Autodesk Inventor part; units mm, degrees
ref_plane "YZ Plane" through (0, 0, 0) normal (1, 0, 0) x (0, 1, 0)
ref_plane "XZ Plane" through (0, 0, 0) normal (0, 1, 0) x (-1, 0, 0)
ref_plane "XY Plane" through (0, 0, 0) normal (0, 0, 1) x (1, 0, 0)
sketch "Sketch1" plane through (0, 0, 0) normal (0, 1, 0) x (-1, 0, 0)
  line L0 (0, 0) -> (1.8, 0)
  line L1 (0, 0) -> (-1.8, 0)
  circle A0 centre (0, 0) radius 2.7
  line L2 (1.8, 0) -> (1.8, 2.0125)
  line L3 (1.8, 0) -> (1.8, -2.0125)
  line L4 (-1.8, 0) -> (-1.8, -2.0125)
  line L5 (-1.8, 0) -> (-1.8, 2.0125)
  circle A1 centre (0, 0) radius 4.7
  dimension "d0" = 1.8
  dimension "d1" = 1.8
  dimension "d2" = 5.4
  dimension "d7" = 9.4
extrude "Extrusion1" add sketch "Sketch1" along normal blind 4 contours L1 L5 A0 L2 L0 | L0 L3 A0 L4 L1 | L2 A0 L3 | L4 A0 L5
extrude "Extrusion2" add sketch "Sketch1" along normal blind 5 from surface at 4 contours L1 L5 A0 L2 L0 | L0 L3 A0 L4 L1
extrude "Extrusion3" add sketch "Sketch1" against normal blind 2 contours L1 L5 A0 L2 L0 | L0 L3 A0 L4 L1 | L2 A0 L3 | L4 A0 L5 | A1
chamfer "Chamfer1" distance 2 angle 45 1 edges at (4.7, 0, 0)
properties part number "driven gear axle"
The listing builds one solid part. Answer for the finished solid, in the listing's coordinates (mm). A direction names the side the tool comes from. Round coordinates to 2 decimals unless told otherwise and drop trailing zeros. Loops run counter-clockwise (first coordinate to the right, second up) from the corner with the lowest first, then second, coordinate; pieces in that order, holes last.
Q1. Find the intervals of material crossed by line 1 (Y direction, x = 2.5, z = -0.5); line 2 (X direction, y = 7, z = -0.5); line 3 (Z direction, x = 0.75, y = 1), in increasing order.
Q2. For a pull along Z with two mould halves and no side action, classify faces 1 (the face through (-2.575, 3.437, -0.811)), 2 (the face through (0, -2, 0)) as released by +Z, released by -Z, zero draft, split by the parting line, or undercut.
Q3. Which of the six approach directions +Z, -Z, +X, -X, +Y, -Y give full straight-line access (tool end or side, diameter ignored) to faces 3 (the face through (1.8, 6, 0)), 4 (the face through (-2, 4, 0)), 5 (the face through (0.613, -0.125, 2.758))?
Q4. Given pin 1 Ø4 at (y, z) = (2, 3.5) entering from -X (3 decimals); pin 2 Ø4.5 at (y, z) = (5.5, 1) entering from -X; pin 3 Ø1.5 at (y, z) = (7.5, 3) entering from -X, each flat-ended and moving along its own axis, determine where each tip first touches the part or whether it passes through.
Q5. Section C-C, the plane y = 1.25 is taken. Determine the outline of the cut face in (x, z), then the cut area to 3 significant figures.
Q6. Section D-D, the plane y = -0.25 is taken. Determine the outline of the cut face in (x, z).
Completed:
1. line 1: y = -2 to 4
1. line 2: x = -1.8 to 1.8
1. line 3: z = -2.59 to 2.59
2. face 1: split by the parting line
2. face 2: zero draft
3. face 3: +Z, -Z, +X, +Y
3. face 4: +Z, -Z, -X, +Y
3. face 5: +Y
4. pin 1: stops at x = -2.245
4. pin 2: stops at x = -2.7
4. pin 3: stops at x = -1.49
5. outline: circle Ø5.4 at (0, 0)
5. area: 22.9 mm2
6. outline: circle Ø5.9 at (0, 0)
